Design review of the part built by this model. Coordinates are the model's own, in mm. Face numbers are marked on the shaded views. A direction names the side the tool comes from. Coordinates: 2 decimals unless noted, no trailing zeros. Order: outer loops, then holes, each group sorted by start corner. A loop starts at its lowest first (then second) coordinate and runs counter-clockwise, first axis right, second up. Notation, with made-up numbers: M 35,8.25 L 64,8.25 A32 ccw 64,34.25 Z; hole C 54.25,5.25 d11. An arc over 180 degrees is marked long. Answer in a Markdown table with one row per item.
from build123d import *

# Parameters (mm, degrees)
F1_DEPTH = 3
F3_DEPTH = 2
F4_DEPTH = 12
F5_START = 12
F5_DEPTH = 2


with BuildPart() as f1:
    # F0 (on Front) → F1 (new body)
    with BuildSketch(Plane.XZ):
        with BuildLine():
            Line((15, 0), (-15, 0))
            ThreePointArc((-15, 0), (0, -15), (15, 0))
        make_face()
    extrude(amount=-F1_DEPTH)

    # F2 (on face) → F3 (join)
    with BuildSketch(Plane.XZ):
        with BuildLine():
            ThreePointArc((-19.5959179423, -4), (-13.408818757, -14.8392580523), (-2, -19.8997487421))
            ThreePointArc((-2, -19.8997487421), (0, -20), (2, -19.8997487421))
            ThreePointArc((2, -19.8997487421), (13.408818757, -14.8392580523), (19.5959179423, -4))
            Line((19.5959179423, -4), (14.4568322948, -4))
            ThreePointArc((14.4568322948, -4), (0, -15), (-14.4568322948, -4))
            Line((-14.4568322948, -4), (-19.5959179423, -4))
        make_face()
        with BuildLine():
            Line((14.4568322948, -4), (-14.4568322948, -4))
            ThreePointArc((-14.4568322948, -4), (0, -15), (14.4568322948, -4))
        make_face()
        with BuildLine():
            ThreePointArc((-20, 0), (-19.8987230601, -2.0101792401), (-19.5959179423, -4))
            Line((-19.5959179423, -4), (-14.4568322948, -4))
            ThreePointArc((-14.4568322948, -4), (-14.8635877974, -2.0183552187), (-15, 0))
            Line((-15, 0), (-20, 0))
        make_face()
        with BuildLine():
            Line((14.4568322948, -4), (19.5959179423, -4))
            ThreePointArc((19.5959179423, -4), (19.8987230601, -2.0101792401), (20, 0))
            Line((20, 0), (15, 0))
            ThreePointArc((15, 0), (14.8635877974, -2.0183552187), (14.4568322948, -4))
        make_face()
        with BuildLine():
            ThreePointArc((-15, 0), (-14.8635877974, -2.0183552187), (-14.4568322948, -4))
            Line((-14.4568322948, -4), (14.4568322948, -4))
            ThreePointArc((14.4568322948, -4), (14.8635877974, -2.0183552187), (15, 0))
            Line((15, 0), (-15, 0))
        make_face()
        with BuildLine():
            Line((-29.7321374946, -4), (-19.5959179423, -4))
            ThreePointArc((-19.5959179423, -4), (-19.8987230601, -2.0101792401), (-20, 0))
            Line((-20, 0), (-30, 0))
            ThreePointArc((-30, 0), (-29.9329594664, -2.0044793789), (-29.7321374946, -4))
        make_face()
        with BuildLine():
            ThreePointArc((20, 0), (19.8987230601, -2.0101792401), (19.5959179423, -4))
            Line((19.5959179423, -4), (29.7321374946, -4))
            ThreePointArc((29.7321374946, -4), (29.9329594664, -2.0044793789), (30, 0))
            Line((30, 0), (20, 0))
        make_face()
        with BuildLine():
            ThreePointArc((2, -19.8997487421), (0, -20), (-2, -19.8997487421))
            Line((-2, -19.8997487421), (-2, -29.9332590942))
            ThreePointArc((-2, -29.9332590942), (0, -30), (2, -29.9332590942))
            Line((2, -29.9332590942), (2, -19.8997487421))
        make_face()
    extrude(amount=F3_DEPTH)

    # F2 (on face) → F4 (join)
    with BuildSketch(Plane.XZ):
        with BuildLine():
            Line((-29.7321374946, -4), (-19.5959179423, -4))
            ThreePointArc((-19.5959179423, -4), (-19.8987230601, -2.0101792401), (-20, 0))
            Line((-20, 0), (-30, 0))
            ThreePointArc((-30, 0), (-29.9329594664, -2.0044793789), (-29.7321374946, -4))
        make_face()
        with BuildLine():
            ThreePointArc((20, 0), (19.8987230601, -2.0101792401), (19.5959179423, -4))
            Line((19.5959179423, -4), (29.7321374946, -4))
            ThreePointArc((29.7321374946, -4), (29.9329594664, -2.0044793789), (30, 0))
            Line((30, 0), (20, 0))
        make_face()
        with BuildLine():
            ThreePointArc((2, -19.8997487421), (0, -20), (-2, -19.8997487421))
            Line((-2, -19.8997487421), (-2, -29.9332590942))
            ThreePointArc((-2, -29.9332590942), (0, -30), (2, -29.9332590942))
            Line((2, -29.9332590942), (2, -19.8997487421))
        make_face()
    extrude(amount=F4_DEPTH)

    # F2 (on face) → F5 (join)
    with BuildSketch(Plane.XZ.offset(F5_START)):
        with BuildLine():
            Line((-2, -29.9332590942), (-2, -19.8997487421))
            ThreePointArc((-2, -19.8997487421), (-13.408818757, -14.8392580523), (-19.5959179423, -4))
            Line((-19.5959179423, -4), (-29.7321374946, -4))
            ThreePointArc((-29.7321374946, -4), (-20.4906227164, -21.9119688913), (-2, -29.9332590942))
        make_face()
        with BuildLine():
            ThreePointArc((19.5959179423, -4), (13.408818757, -14.8392580523), (2, -19.8997487421))
            Line((2, -19.8997487421), (2, -29.9332590942))
            ThreePointArc((2, -29.9332590942), (20.4906227164, -21.9119688913), (29.7321374946, -4))
            Line((29.7321374946, -4), (19.5959179423, -4))
        make_face()
        with BuildLine():
            Line((-29.7321374946, -4), (-19.5959179423, -4))
            ThreePointArc((-19.5959179423, -4), (-19.8987230601, -2.0101792401), (-20, 0))
            Line((-20, 0), (-30, 0))
            ThreePointArc((-30, 0), (-29.9329594664, -2.0044793789), (-29.7321374946, -4))
        make_face()
        with BuildLine():
            ThreePointArc((2, -19.8997487421), (0, -20), (-2, -19.8997487421))
            Line((-2, -19.8997487421), (-2, -29.9332590942))
            ThreePointArc((-2, -29.9332590942), (0, -30), (2, -29.9332590942))
            Line((2, -29.9332590942), (2, -19.8997487421))
        make_face()
        with BuildLine():
            ThreePointArc((20, 0), (19.8987230601, -2.0101792401), (19.5959179423, -4))
            Line((19.5959179423, -4), (29.7321374946, -4))
            ThreePointArc((29.7321374946, -4), (29.9329594664, -2.0044793789), (30, 0))
            Line((30, 0), (20, 0))
        make_face()
    extrude(amount=F5_DEPTH)


solid = f1.part
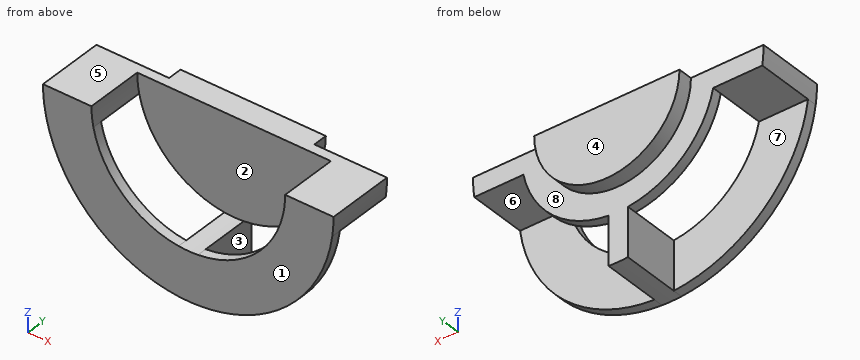
(1) For the marked faces 4, 5, 6, 7 and 8, list the 3-axis set-ups (+Z, -Z, +X, -X, +Y, -Y) from which the entire face can be reached by the end or side of a thin tool; tool diameter is ignored.
Return value:
| item | result |
|---|---|
| face 4 | +Z, -Z, +X, -X, +Y |
| face 5 | +Z, +X, -X, +Y, -Y |
| face 6 | -Z, +X, +Y |
| face 7 | -Z, -X, +Y |
| face 8 | -Z, +Y |
(2) Add section B-B, the plane z = -10. Give the boundary of the cut face in (x, y).
Return value:
| item | result |
|---|---|
| outline | M -28.28,-14 L -17.32,-14 L -17.32,-12 L -28.28,-12 Z; M -17.32,-2 L 17.32,-2 L 17.32,0 L 11.18,0 L 11.18,3 L -11.18,3 L -11.18,0 L -17.32,0 Z; M 17.32,-14 L 28.28,-14 L 28.28,-12 L 17.32,-12 Z |
(3) Add section C-C, the plane x = 9.5. Give the boundary of the cut face in (y, z), and give its area (3 significant figures).
Return value:
| item | result |
|---|---|
| outline | M -14,-28.46 L -12,-28.46 L -12,-17.6 L -14,-17.6 Z; M -2,-17.6 L 0,-17.6 L 0,-11.61 L 3,-11.61 L 3,0 L -2,0 Z |
| area | 91.7 mm2 |
(4) Insertion check: pin 1 Ø2 at (y, z) = (0.5, -9) entering from -X; pin 2 Ø1 at (x, z) = (0.5, -15) entering from -Y; pin 3 Ø9 at (x, z) = (15, -19.5) entering from +Y. Each pin has a flat end and moves straight along its axis. Give the tip position at first contact, or say it passes through.
Return value:
| item | result |
|---|---|
| pin 1 | stops at x = -18.27 |
| pin 2 | stops at y = -2 |
| pin 3 | stops at y = -12 |
(5) Add section D-D, the plane x = 0. Give the boundary of the cut face in (y, z), and give its area (3 significant figures).
Return value:
| item | result |
|---|---|
| outline | M -14,-30 L 0,-30 L 0,-15 L 3,-15 L 3,0 L -2,0 L -2,-20 L -14,-20 Z |
| area | 225 mm2 |
(6) For line 1 along Y through (x, z) = (-20, -13); line 2 along Z through (x, y) = (23, -11); line 3 along Z through (x, y) = (0, -10.5), list the stretches that pass through material, from the lowest coordinate up. Write a range as from..to.
Return value:
| item | result |
|---|---|
| line 1 | y = -14..-12 |
| line 2 | z = -4..0 |
| line 3 | z = -30..-20 |
(7) Draft analysis for pull direction X (two halves, no side actions). For the marked faces 1, 2 and 3, state which applies: pulls with the +X half, pulls with the -X half, needs draft (parallel to the pull), parting line crosses it, or undercut.
Return value:
| item | result |
|---|---|
| face 1 | needs draft |
| face 2 | undercut |
| face 3 | pulls with the +X half |
(8) Add section A-A, the plane y = -4.25. Give the boundary of the cut face in (x, z), and give its area (3 significant figures).
Return value:
| item | result |
|---|---|
| outline | M -30,0 A30 ccw -29.73,-4 L -19.6,-4 A20 cw -20,0 Z; M -2,-29.93 A30 ccw 2,-29.93 L 2,-19.9 A20 cw -2,-19.9 Z; M 19.6,-4 L 29.73,-4 A30 ccw 30,0 L 20,0 A20 cw Z |
| area | 120 mm2 |
